Can you work these out from the model? Positions are in its coordinate system, mm. Round coordinates to 2 decimals unless told otherwise and drop trailing zeros. Order: outer loops, then holes, each group sorted by start corner. A loop starts at its lowest first (then second) coordinate and runs counter-clockwise, first axis right, second up.
Q1. Will these pins go through, and if not, where does the flat tip stop? P1, Ø1, axis at y = -105, z = 6.5, coming from the +X side; P2, Ø4.5, axis at y = 95.5, z = 8, coming from the -X side; P3, Ø2, axis at y = -45, z = 11.5, coming from the -X side.
Q2. If I drill on line 1 (Y direction, x = -153.5, z = 3); line 2 (X direction, y = -107.5, z = 1.75); line 3 (X direction, y = 51, z = 13), over which ranges is the centre line in solid material (lowest first)?
Q3. If we section it at B-B (y = 105.5): Please give me the cut outline in (x, z), plus the area to 3 significant figures.
Q4. If we section it at A-A (x = 150.5): Please give me the cut outline in (y, z), plus the area to 3 significant figures.
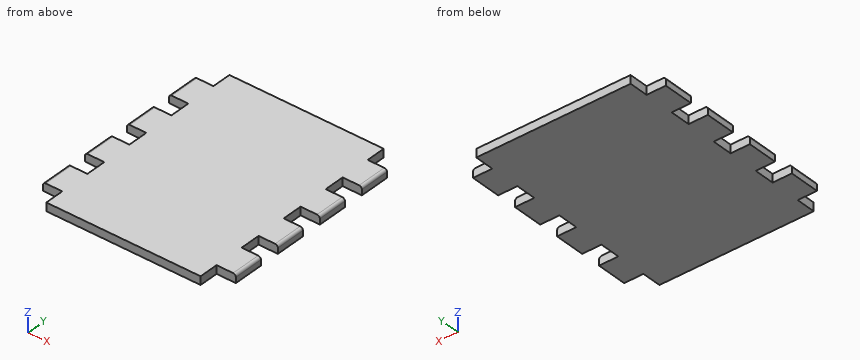
from build123d import *

# Parameters (mm, degrees)
F1_DEPTH = 15
F3_R     = 5


with BuildPart() as f1:
    # F0 (on Top) → F1 (new body)
    with BuildSketch(Plane.XY):
        Polygon((-140, 165.5), (-175, 165.5), (-175, 110.5), (-140, 110.5), (-140, 73.5), (-175, 73.5), (-175, 18.5), (-140, 18.5), (-140, 0), (0, 0), (0, 200.5), (-140, 200.5), align=None)
    extrude(amount=F1_DEPTH)

    # F2: F1 across plane


with BuildPart() as f1_1:
    add(f1.part)
    add(f1.part.mirror(Plane.XZ))

    # F3
    f3_edges = [f1_1.edges().sort_by_distance(p)[0] for p in [
        (-175, 138, 15),
        (-175, 46, 15),
        (-175, -46, 15),
        (-175, -138, 15),
    ]]
    fillet(f3_edges, radius=F3_R)

    # F4: F1 across face


with BuildPart() as f1_2:
    add(f1_1.part)
    add(f1_1.part.mirror(Plane(origin=(0, 0, 7.5), x_dir=(0, 1, 0), z_dir=(1, 0, 0))))


solid = f1_2.part
Solution:
1. P1: stops at x = 140
1. P2: stops at x = -140
1. P3: stops at x = -174.97
2. line 1: y = -165.5 to -110.5, -73.5 to -18.5, 18.5 to 73.5, 110.5 to 165.5
2. line 2: x = -140 to 140
2. line 3: x = -174 to 174
3. outline: (-140, 0) - (140, 0) - (140, 15) - (-140, 15) - close
3. area: 4,200 mm2
4. outline: (-165.5, 0) - (-110.5, 0) - (-110.5, 15) - (-165.5, 15) - close; (-73.5, 0) - (-18.5, 0) - (-18.5, 15) - (-73.5, 15) - close; (18.5, 0) - (73.5, 0) - (73.5, 15) - (18.5, 15) - close; (110.5, 0) - (165.5, 0) - (165.5, 15) - (110.5, 15) - close
4. area: 3,300 mm2
